For this review, take the finished solid that the model builds, in its own axes (mm). Face numbers are marked on the shaded views. Coordinates: 2 decimals unless noted, no trailing zeros. Loops run counter-clockwise (first coordinate to the right, second up) from the corner with the lowest first, then second, coordinate; pieces in that order, holes last. Notation, with made-up numbers: M -33,37.25 L -17,37.25 A24 cw -17,69.25 Z; hole C -30,-27 d4. An arc over 180 degrees is marked long. Use one line per item in the form item = value.
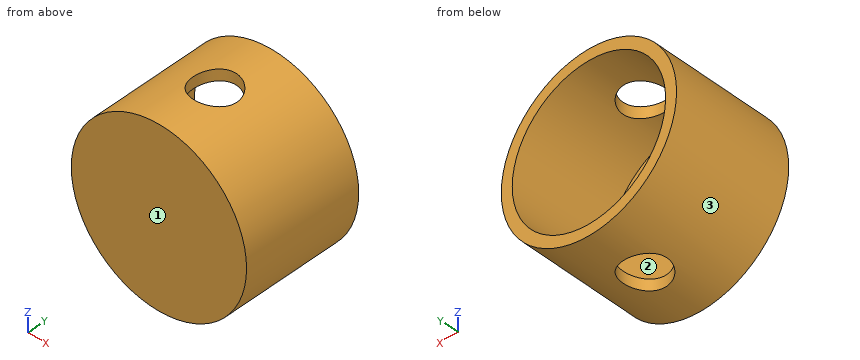
```python
from build123d import *

# Parameters (mm, degrees)
F0_R      = 50.8
F1_DEPTH  = 35
F2_R      = 44.45
F3_DEPTH  = 82.563922
F3_FACE_R = 44.45
F4_DEPTH  = 25.4
F5_R      = 12.7
F6_DEPTH  = 71.218602


with BuildPart() as f1:
    # F0 (on Front) → F1 (new body, symmetric)
    with BuildSketch(Plane.XZ):
        Circle(F0_R)
    extrude(amount=F1_DEPTH, both=True)

    # F2 (on Front) → F3 (cut)
    with BuildSketch(Plane.XZ):
        Circle(F2_R)
    extrude(amount=-F3_DEPTH, mode=Mode.SUBTRACT)

    # F3_face (on face) → F4 (cut)
    with BuildSketch(Plane(origin=(0, 0, 0), x_dir=(1, 0, 0), z_dir=(0, 1, 0))):
        Circle(F3_FACE_R)
    extrude(amount=-F4_DEPTH, mode=Mode.SUBTRACT)

    # F5 (on Top) → F6 (cut, symmetric)
    with BuildSketch(Plane.XY):
        Circle(F5_R)
    extrude(amount=F6_DEPTH, both=True, mode=Mode.SUBTRACT)


solid = f1.part
```
1. Consider section D-D on x = 21. Write out the cut boundary in (y, z), plus the area to 3 significant figures.
Computed values:
outline = M -35,-46.26 L 35,-46.26 L 35,-39.18 L -25.4,-39.18 L -25.4,39.18 L 35,39.18 L 35,46.26 L -35,46.26 Z
area = 1,740 mm2
2. Consider section A-A on x = 0. Write out the cut boundary in (y, z).
Computed values:
outline = M -35,-50.8 L -12.7,-50.8 L -12.7,-44.45 L -25.4,-44.45 L -25.4,44.45 L -12.7,44.45 L -12.7,50.8 L -35,50.8 Z; M 12.7,-50.8 L 35,-50.8 L 35,-44.45 L 12.7,-44.45 Z; M 12.7,44.45 L 35,44.45 L 35,50.8 L 12.7,50.8 Z
3. Draft analysis for pull direction Z (two halves, no side actions). For the marked faces 1, 2 and 3, state which applies: +Z half, -Z half, draft (parallel to the pull), parting line (faces both ways), or undercut.
Computed values:
face_1 = draft
face_2 = undercut
face_3 = parting line
4. Consider section C-C on z = 0. Write out the cut boundary in (x, y), plus the area to 3 significant figures.
Computed values:
outline = M -50.8,-35 L 50.8,-35 L 50.8,35 L 44.45,35 L 44.45,-25.4 L -44.45,-25.4 L -44.45,35 L -50.8,35 Z
area = 1,740 mm2
5. Consider section B-B on y = 2. Write out the cut boundary in (x, z), plus the area to 3 significant figures.
Computed values:
outline = M -12.54,-49.23 L -12.54,-42.64 A44.45 cw -12.54,42.64 L -12.54,49.23 A50.8 ccw Z; M 12.54,-49.23 A50.8 ccw 12.54,49.23 L 12.54,42.64 A44.45 cw 12.54,-42.64 Z
area = 1,580 mm2
6. Wall thickness on line 1 along Y through (x, z) = (0, 44.5); line 2 along Y through (x, z) = (-3, -38); line 3 along Z through (x, y) = (-12, 9): over which ranges is each line inside the solid? List them lowest first. Write a range as from..to.
Computed values:
line_1 = -35..-12.7, 12.7..35
line_2 = -35..-25.4
line_3 = -49.36..-42.8, 42.8..49.36
7. For pin 1 Ø10 at (y, z) = (16.5, 32.5) entering from -X; pin 2 Ø10 at (x, y) = (16.5, -11) entering from -Z; pin 3 Ø1 at (x, z) = (-39, -6.5) entering from +Y, all flat-tipped, find the tip position at first contact; note any pin that passes through.
Computed values:
pin_1 = -42.71
pin_2 = -49.48
pin_3 = -25.4
